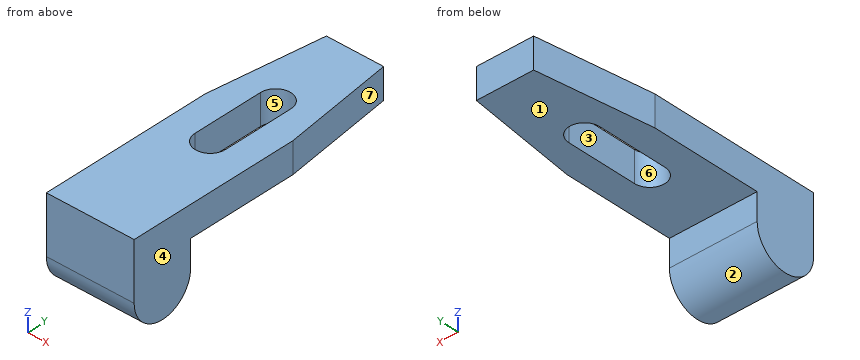
```python
from build123d import *

# Parameters (mm, degrees)
F1_DEPTH = 46
F3_DEPTH = 25
F5_DEPTH = 25


with BuildPart() as f1:
    # F0 (on Right) → F1 (new body)
    with BuildSketch(Plane.YZ):
        with BuildLine():
            Line((76.981132, -29.915097), (76.981132, -13.915097))
            Line((76.981132, -13.915097), (-41.018868, -13.915097))
            Line((-41.018868, -13.915097), (-73.018868, -13.915097))
            Line((-73.018868, -13.915097), (-73.018868, -29.915097))
            Line((-73.018868, -29.915097), (-73.018868, -43.915097))
            ThreePointArc((-73.018868, -43.915097), (-57.018868, -59.915097), (-41.018868, -43.915097))
            Line((-41.018868, -43.915097), (-41.018868, -29.915097))
            Line((-41.018868, -29.915097), (76.981132, -29.915097))
        make_face()
    extrude(amount=F1_DEPTH)

    # F2 (on face) → F3 (cut)
    with BuildSketch(Plane.XY.offset(-13.915097)):
        Polygon((46, 76.981132), (38, 76.981132), (46, 16.981132), align=None)
        Polygon((0, 16.981132), (7.994875, 76.981132), (0, 76.981132), align=None)
    extrude(amount=-F3_DEPTH, mode=Mode.SUBTRACT)

    # F4 (on face) → F5 (cut)
    with BuildSketch(Plane.XY.offset(-13.915097)):
        with BuildLine():
            ThreePointArc((31, 31.981132), (23, 39.981132), (15, 31.981132))
            Line((15, 31.981132), (15, -5.018868))
            ThreePointArc((15, -5.018868), (23, -13.018868), (31, -5.018868))
            Line((31, -5.018868), (31, 31.981132))
        make_face()
    extrude(amount=-F5_DEPTH, mode=Mode.SUBTRACT)


solid = f1.part
```
CAD build for the part. Positions are in the model's coordinates, mm. Face numbers are marked on the shaded views. A direction names the side the tool comes from. Round coordinates to 2 decimals unless told otherwise and drop trailing zeros. Write each loop counter-clockwise with the first axis right and the second up, starting at its lowest first coordinate (ties: lowest second). Pieces come first, ordered by that corner, then holes.
Item 1: Drop flat-ended pins along their axis: pin 1 Ø3 at (x, z) = (11, -47.5) entering from -Y; pin 2 Ø8 at (y, z) = (21, -24) entering from +X; pin 3 Ø10 at (x, z) = (17.5, -53.5) entering from -Y. Give the stop position or say it passes through.
Filled in:
pin 1: stops at y = -72.88
pin 2: stops at x = 46
pin 3: stops at y = -72.35
Item 2: Tool access for the marked faces 1, 2 and 3: list every direction of +Z, -Z, +X, -X, +Y, -Y with a clear straight run to the whole face (end or side of a thin tool).
Filled in:
face 1: -Z, +X, -X, +Y
face 2: -Z, +X, -X
face 3: +Z, -Z
Item 3: Mould opens along Y. For the marked faces 4, 5, 6 and 7 say: released by +Y, released by -Y, zero draft, split by the parting line, or undercut.
Filled in:
face 4: zero draft
face 5: undercut
face 6: undercut
face 7: released by +Y
Item 4: Band-saw the part on A-A on x = 23. Write the cut outline in (y, z), then the cut area to 3 significant figures.
Filled in:
outline: (-73.02, -43.92) arc R16 ccw to (-41.02, -43.92) - (-41.02, -29.92) - (-13.02, -29.92) - (-13.02, -13.92) - (-73.02, -13.92) - close; (39.98, -29.92) - (76.98, -29.92) - (76.98, -13.92) - (39.98, -13.92) - close
area: 2,400 mm2
Item 5: Band-saw the part on C-C on z = -34. Write the cut outline in (x, y), then the cut area to 3 significant figures.
Filled in:
outline: (0, -73.02) - (46, -73.02) - (46, -41.02) - (0, -41.02) - close
area: 1,470 mm2
Item 6: Band-saw the part on D-D on x = 42. Write the cut outline in (y, z), then the cut area to 3 significant figures.
Filled in:
outline: (-73.02, -43.92) arc R16 ccw to (-41.02, -43.92) - (-41.02, -29.92) - (46.98, -29.92) - (46.98, -13.92) - (-73.02, -13.92) - close
area: 2,770 mm2
Item 7: Drill centre lines: L1, parallel to Y at x = 13, z = -32.5; L2, parallel to Z at x = 24.5, y = -27; L3, parallel to Y at x = 16, z = -26. Where is each one in solid material? Low to high.
Filled in:
L1: y = -73.02 to -41.02
L2: z = -29.92 to -13.92
L3: y = -73.02 to -8.89, 35.85 to 76.98
Item 8: Band-saw the part on B-B on y = 27. Write the cut outline in (x, z) (3 decimals), then the cut area to 3 significant figures.
Filled in:
outline: (1.335, -29.915) - (15, -29.915) - (15, -13.915) - (1.335, -13.915) - close; (31, -29.915) - (44.664, -29.915) - (44.664, -13.915) - (31, -13.915) - close
area: 437 mm2
